from build123d import *

# Parameters (mm, degrees)
SKETCH_1_W          = 24
SKETCH_1_H          = 15
EXTRUDE_1_DEPTH     = 4
SKETCH_2_W          = 24
SKETCH_2_H          = 4
EXTRUDE_2_DEPTH     = 11
SKETCH_3_R          = 1.25
CUT_EXTRUDE_1_DEPTH = 5
SKETCH_4_R          = 1.25
CUT_EXTRUDE_2_DEPTH = 5


with BuildPart() as part:
    # 草图1 → 凸台-拉伸1 (new body)
    with BuildSketch(Plane.XY):
        Rectangle(SKETCH_1_W, SKETCH_1_H)
    extrude(amount=EXTRUDE_1_DEPTH)

    # 草图2 → 凸台-拉伸2 (add)
    with BuildSketch(Plane.XY.offset(4)):
        with Locations((0, 5.5)):
            Rectangle(SKETCH_2_W, SKETCH_2_H)
    extrude(amount=EXTRUDE_2_DEPTH)

    # 草图3 → 切除-拉伸1 (cut, through all)
    with BuildSketch(Plane.XY.offset(4)):
        with Locations((-9, -2.5)):
            Circle(SKETCH_3_R)
        with Locations((9, -2.5)):
            Circle(SKETCH_3_R)
    extrude(amount=-CUT_EXTRUDE_1_DEPTH, mode=Mode.SUBTRACT)

    # 草图4 → 切除-拉伸2 (cut, through all)
    with BuildSketch(Plane.XZ.offset(-3.5)):
        with Locations((-4.5, 10)):
            Circle(SKETCH_4_R)
        with Locations((4.5, 10)):
            Circle(SKETCH_4_R)
    extrude(amount=-CUT_EXTRUDE_2_DEPTH, mode=Mode.SUBTRACT)


solid = part.part
Verification items for the finished model (mm, model axes). A direction names the side the tool comes from. Coordinates: 2 decimals unless noted, no trailing zeros. Order: outer loops, then holes, each group sorted by start corner. A loop starts at its lowest first (then second) coordinate and runs counter-clockwise, first axis right, second up.
Item 1: Release check for a two-part mould opening along Y. For faces 1 (the face through (0, 7.5, 7)), 2 (the face through (7.75, -2.45, 2.03)), 3 (the face through (-10.25, -2.45, 2.03)), 4 (the face through (0, 0, 0)) record: +Y half, -Y half, draft (parallel to the pull), parting line (faces both ways), or undercut.
Filled in:
face 1: +Y half
face 2: undercut
face 3: undercut
face 4: draft
Item 2: Section check A-A, the plane z = 10. Enter the section's corners in (x, y).
Filled in:
outline: (-12, 3.5) - (-5.75, 3.5) - (-5.75, 7.5) - (-12, 7.5) - close; (-3.25, 3.5) - (3.25, 3.5) - (3.25, 7.5) - (-3.25, 7.5) - close; (5.75, 3.5) - (12, 3.5) - (12, 7.5) - (5.75, 7.5) - close
Item 3: Section check C-C, the plane y = -2.5. Enter the section's corners in (x, z).
Filled in:
outline: (-12, 0) - (-10.25, 0) - (-10.25, 4) - (-12, 4) - close; (-7.75, 0) - (7.75, 0) - (7.75, 4) - (-7.75, 4) - close; (10.25, 0) - (12, 0) - (12, 4) - (10.25, 4) - close
Item 4: Section check D-D, the plane x = 7.25. Enter the section's corners in (y, z).
Filled in:
outline: (-7.5, 0) - (7.5, 0) - (7.5, 15) - (3.5, 15) - (3.5, 4) - (-7.5, 4) - close
Item 5: Section check B-B, the plane x = 4.5. Enter the section's corners in (y, z).
Filled in:
outline: (-7.5, 0) - (7.5, 0) - (7.5, 8.75) - (3.5, 8.75) - (3.5, 4) - (-7.5, 4) - close; (3.5, 11.25) - (7.5, 11.25) - (7.5, 15) - (3.5, 15) - close
Item 6: Material ranges on L1, parallel to Y at x = -9, z = 1.05; L2, parallel to Y at x = -4.5, z = 6.5; L3, parallel to Z at x = 2.5, y = -5, recorded low to high.
Filled in:
L1: y = -7.5 to -3.75, -1.25 to 7.5
L2: y = 3.5 to 7.5
L3: z = 0 to 4
Item 7: Access from +Z, -Z, +X, -X, +Y, -Y to the whole of each face (thin tool, end or side, straight path). Record for faces 5 (the face through (-12, 3, 2)), 6 (the face through (0, 3.5, 9)).
Filled in:
face 5: +Z, -Z, -X, +Y, -Y
face 6: +Z, +X, -X, -Y
Item 8: Depth check by flat-ended pin: pin 1 (2 mm diameter, centred on x = 9, y = -2.5, fed in from -Z); pin 2 (5.5 mm diameter, centred on x = 2.5, y = -2, fed in from +Z); pin 3 (4 mm diameter, centred on x = -4.5, z = 10, fed in from +Y); pin 4 (3.5 mm diameter, centred on x = 5.5, z = 9, fed in from -Y). Enter the tip coordinate at first touch or a pass-through.
Filled in:
pin 1: passes through
pin 2: stops at z = 4
pin 3: stops at y = 7.5
pin 4: stops at y = 3.5
